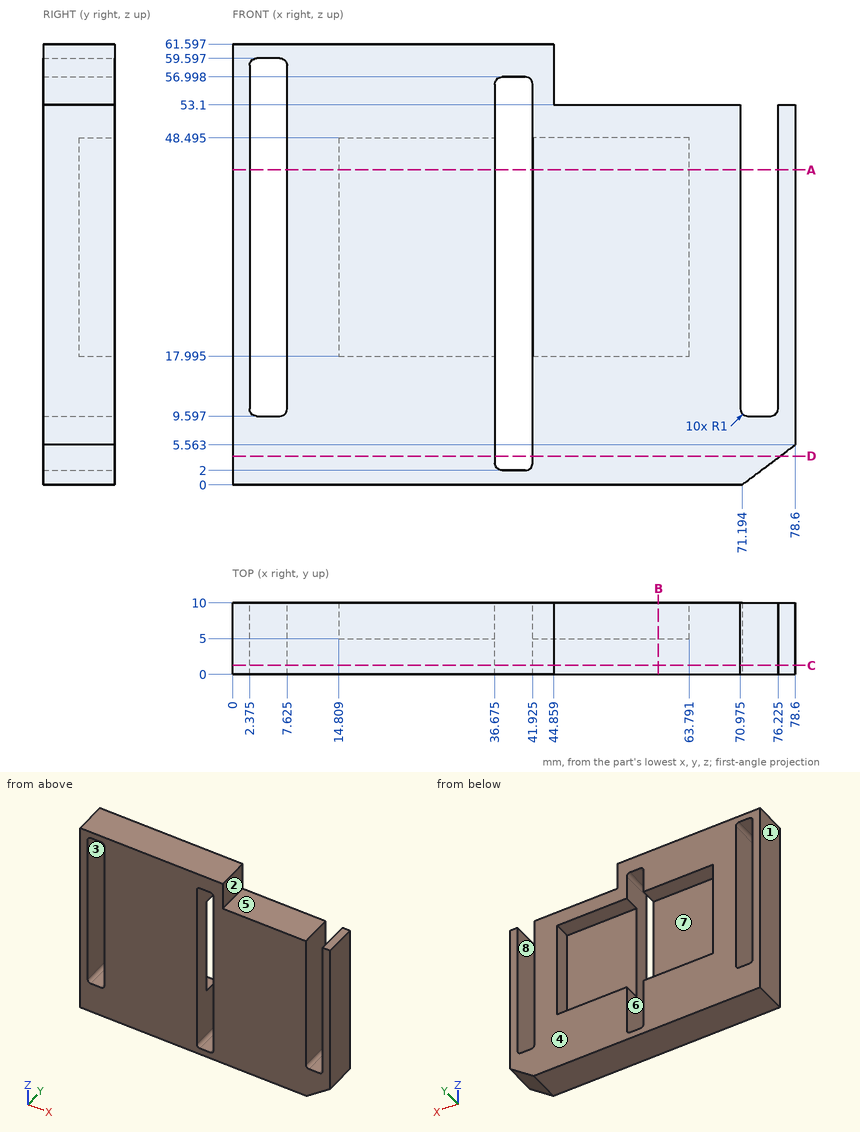
Input: dimensioned drawing with shaded views. Units: mm. Origin: part minimum x, y, z. A direction names the side the tool comes from. Give positions to 0.01 mm unless a question says otherwise; leave off trailing zeros. Write each loop counter-clockwise with the first axis right and the second up, starting at its lowest first coordinate (ties: lowest second). Pieces come first, ordered by that corner, then holes. Notation, with made-up numbers: M 44.5,83.5 L 75.5,83.5 A14 ccw 75.5,91.5 Z; hole C -12,20 d8. An arc over 180 degrees is marked long. Return JSON: item names as keys, results as strings. Group by question number.
1) Pin query (flat end, axial travel): P1, Ø1.9, axis at x = 78, y = 4.5, coming from the +Z side; P2, Ø1, axis at x = 73.5, y = 3, coming from the +Z side. Return the tip coordinate at first contact, or that it passes through.
2) Set-up query: the marked faces 5, 6, 7 and 8. Return all of +Z, -Z, +X, -X, +Y, -Y with unobstructed straight access to the full face (end or side cutting, diameter ignored); none if empty.
3) Cut plane C-C, the plane y = 1.25. Give the number of separate pieces and of enclosed holes in the cut face, plus the area to 3 significant figures.
4) Cut plane B-B, the plane x = 59.5. Output: boundary loops of the cut face in (y, z) (1 decimal).
5) Material intervals for line 1 along X through (y, z) = (8.5, 52) (1 decimal); line 2 along X through (y, z) = (6.25, 37.5) (1 decimal); line 3 along X through (y, z) = (1.75, 55.5) (1 decimal), sorted ascending. Write a range as [from, to].
6) Pull-direction query (X, two-part tool) for the marked faces 1, 2, 3 and 4; classes: pulls with the +X half, pulls with the -X half, needs draft (parallel to the pull), parting line crosses it, or undercut.
7) Cut plane A-A, the plane z = 44. Output: boundary loops of the cut face in (x, y) (1 decimal).
8) Cut plane D-D, the plane z = 4. Output: boundary loops of the cut face in (x, y) (1 decimal), plus the area to 3 significant figures.
Recorded:
{
 "1": {"P1": "stops at z = 53.1", "P2": "stops at z = 9.6"},
 "2": {"face 5": "+Z, +X, +Y, -Y", "face 6": "+Y, -Y", "face 7": "+Y", "face 8": "+Z, +Y, -Y"},
 "3": {"separate pieces": "1", "enclosed holes": "2", "area": "3,760 mm²"},
 "4": {"outline": "M 0,0 L 10,0 L 10,18 L 5,18 L 5,48.5 L 10,48.5 L 10,53.1 L 0,53.1 Z"},
 "5": {"line 1": "x = [0, 2.4], [7.6, 36.7], [41.9, 71], [76.2, 78.6]", "line 2": "x = [0, 2.4], [7.6, 14.8], [63.8, 71], [76.2, 78.6]", "line 3": "x = [0, 2.4], [7.6, 36.7], [41.9, 44.9]"},
 "6": {"face 1": "pulls with the -X half", "face 2": "pulls with the +X half", "face 3": "undercut", "face 4": "needs draft"},
 "7": {"outline": "M 0,0 L 2.4,0 L 2.4,10 L 0,10 Z; M 7.6,0 L 36.7,0 L 36.7,5 L 14.8,5 L 14.8,10 L 7.6,10 Z; M 41.9,0 L 71,0 L 71,10 L 63.8,10 L 63.8,5 L 41.9,5 Z; M 76.2,0 L 78.6,0 L 78.6,10 L 76.2,10 Z"},
 "8": {"outline": "M 0,0 L 36.7,0 L 36.7,10 L 0,10 Z; M 41.9,0 L 76.5,0 L 76.5,10 L 41.9,10 Z", "area": "713 mm²"}
}
